```python
from build123d import *

# Parameters (mm, degrees)
BOSS_EXTRUDE1_DEPTH = 38
SKETCH2_R           = 5
SKETCH2_R_2         = 1.6
CUT_EXTRUDE1_DEPTH  = 47.540305113
SKETCH3_R           = 2.6
CUT_EXTRUDE2_DEPTH  = 46.760244755
FILLET1_R           = 1


with BuildPart() as part:
    # Sketch1 → Boss-Extrude1 (new body)
    with BuildSketch(Plane.XY):
        Polygon((0, 0), (0, -19), (-2, -19), (-2, -2), (-19, -2), (-19, 0), align=None)
    extrude(amount=BOSS_EXTRUDE1_DEPTH)

    # Sketch2 → Cut-Extrude1 (cut, through all)
    with BuildSketch(Plane(origin=(0, 0, 0), x_dir=(0, 0, -1), z_dir=(1, 0, 0))):
        with Locations(Location((-19, -11, 0), (0, 0, 90))):
            Circle(SKETCH2_R)
        with Locations(Location((-27, -11, 0), (0, 0, 90))):
            Circle(SKETCH2_R_2)
        with Locations((-11, -11)):
            Circle(SKETCH2_R_2)
    extrude(amount=-CUT_EXTRUDE1_DEPTH, mode=Mode.SUBTRACT)

    # Sketch3 → Cut-Extrude2 (cut, through all)
    with BuildSketch(Plane.XZ.offset(2)):
        with Locations((-10.5, 34)):
            Circle(SKETCH3_R)
        with Locations(Location((-10.5, 4, 0), (0, 0, 180))):
            Circle(SKETCH3_R)
    extrude(amount=-CUT_EXTRUDE2_DEPTH, mode=Mode.SUBTRACT)

    # Fillet1
    fillet1_edges = [part.edges().sort_by_distance(p)[0] for p in [
        (-1, -19, 38),
        (-1, -19, 0),
        (-19, -1, 38),
        (-19, -1, 0),
    ]]
    fillet(fillet1_edges, radius=FILLET1_R)


solid = part.part
```
Geometry check sheet. Reference: the model listing, model coordinates, mm. A direction names the side the tool comes from. Coordinates: 2 decimals unless noted, no trailing zeros. Loops run counter-clockwise (first coordinate to the right, second up) from the corner with the lowest first, then second, coordinate; pieces in that order, holes last. Notation, with made-up numbers: (49.25, -27.5) - (71.25, -27.5) arc R17 ccw to (71.25, -5.5) - close; hole circle Ø10 at (51.25, 33.25). An arc over 180 degrees is marked (long way). One line per item, written item: value. Start each with the question number.
(1) Mould release check, pull along Y, two halves, no side actions. Record for faces 1 (the flat face through (-19, -1, 19)), 2 (the cylindrical face through (-0.986, -8.693, 14.564)), 3 (the cylindrical face through (-1.014, -18.699, 37.715)): released by +Y, released by -Y, zero draft, split by the parting line, or undercut.
(2) Cross-section at B-B on z = 11. Enter the section's corners in (x, y), plus the area to 3 significant figures.
(3) Tool access check on faces 4 (the cylindrical face through (-18.699, -0.986, 0.285)), 5 (the flat face through (-10, -2, 19)). Record the directions out of +Z, -Z, +X, -X, +Y, -Y that give a thin tool (end or side, any length) a straight path to the whole face; none if there is none.
(4) Material ranges on line 1 (X direction, y = -14.5, z = 26); line 2 (X direction, y = -1.5, z = 4); line 3 (Z direction, x = -1.5, y = -14.25), recorded low to high. Write a range as [from, to].
(5) Depth check by flat-ended pin: P1, Ø8.5, axis at x = -7.5, z = 11, coming from the -Y side; P2, Ø2, axis at y = -14, z = 33.5, coming from the +X side; P3, Ø5, axis at y = -11, z = 11, coming from the -X side. Enter the tip coordinate at first touch or a pass-through.
(6) Cross-section at A-A on x = -10.5. Enter the section's corners in (y, z).
(7) Cross-section at D-D on z = 15. Enter the section's corners in (x, y).
(8) Cross-section at C-C on y = -11. Enter the section's corners in (x, z), plus the area to 3 significant figures.
Results below:
1. face 1: zero draft
1. face 2: undercut
1. face 3: released by -Y
2. outline: (-19, -2) - (-2, -2) - (-2, -9.4) - (0, -9.4) - (0, 0) - (-19, 0) - close; (-2, -19) - (0, -19) - (0, -12.6) - (-2, -12.6) - close
2. area: 65.6 mm2
3. face 4: -Z, -X, +Y, -Y
3. face 5: +Z, -Z, -X, -Y
4. line 1: x = [-2, 0]
4. line 2: x = [-19, -13.1], [-7.9, 0]
4. line 3: z = [0, 15.2], [22.8, 38]
5. P1: stops at y = -2
5. P2: stops at x = 0
5. P3: stops at x = -2
6. outline: (-2, 0) - (0, 0) - (0, 1.4) - (-2, 1.4) - close; (-2, 6.6) - (0, 6.6) - (0, 31.4) - (-2, 31.4) - close; (-2, 36.6) - (0, 36.6) - (0, 38) - (-2, 38) - close
7. outline: (-19, -2) - (-2, -2) - (-2, -8) - (0, -8) - (0, 0) - (-19, 0) - close; (-2, -19) - (0, -19) - (0, -14) - (-2, -14) - close
8. outline: (-2, 0) - (0, 0) - (0, 9.4) - (-2, 9.4) - close; (-2, 12.6) - (0, 12.6) - (0, 14) - (-2, 14) - close; (-2, 24) - (0, 24) - (0, 25.4) - (-2, 25.4) - close; (-2, 28.6) - (0, 28.6) - (0, 38) - (-2, 38) - close
8. area: 43.2 mm2
